from build123d import *

# Parameters (mm, degrees)
SKETCH2_R           = 7.62
BOSS_EXTRUDE2_DEPTH = 254
SKETCH3_R           = 5.08
CUT_EXTRUDE1_DEPTH  = 8.62


with BuildPart() as part:
    # Sketch2 → Boss-Extrude2 (new body)
    with BuildSketch(Plane(origin=(0, 0, 0), x_dir=(1, 0, 0), z_dir=(0, 1, 0))):
        Circle(SKETCH2_R)
    extrude(amount=BOSS_EXTRUDE2_DEPTH)

    # Sketch3 → Cut-Extrude1 (cut, through all)
    with BuildSketch(Plane(origin=(0, 0, 0), x_dir=(0, 0, -1), z_dir=(1, 0, 0))):
        with Locations((0, 157.537141192)):
            Circle(SKETCH3_R)
        with Locations((0, 81.337141192)):
            Circle(SKETCH3_R)
    extrude(amount=-CUT_EXTRUDE1_DEPTH, mode=Mode.SUBTRACT)


solid = part.part
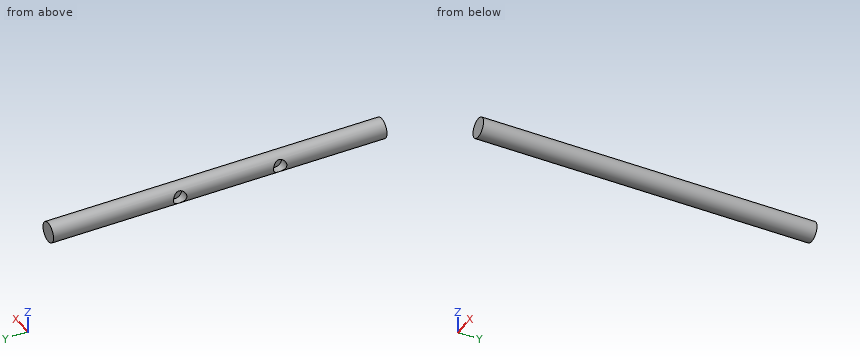
Check sheet for the modelled part. Datum: model origin and axes. Units: mm. Round coordinates to 2 decimals unless told otherwise and drop trailing zeros. Order: outer loops, then holes, each group sorted by start corner. A loop starts at its lowest first (then second) coordinate and runs counter-clockwise, first axis right, second up. Notation, with made-up numbers: M 61,72 L 67,72 A30 cw 67,101 Z; hole C 27,14.5 d8. An arc over 180 degrees is marked long. One line per item, written item: value. Start each with the question number.
1. Section check A-A on z = 0. Enter the section's corners in (x, y), and give its area (3 significant figures).
2. Section check C-C on x = 5. Enter the section's corners in (y, z), and give its area (3 significant figures).
3. Gauge pin test, flat ends, axial feed: P1, Ø8, axis at x = -5.5, y = 96.5, coming from the +Z side; P2, Ø6, axis at y = 157.54, z = 0, coming from the -X side; P3, Ø1, axis at x = -3.5, z = -1, coming from the -Y side; P4, Ø1, axis at y = 84, z = -4.5, coming from the -X side. Record the tip position at first contact, or that the pin passes through.
4. Section check B-B on y = 141.5. Enter the section's corners in (x, z), and give its area (3 significant figures).
5. Scan lines: line 1 along Y through (x, z) = (-4, 0); line 2 along Y through (x, z) = (-6, 1.75); line 3 along Z through (x, y) = (-3.25, 79). Record each from-to range of solid material in increasing order.
Results found:
1. outline: M -7.62,0 L 7.62,0 L 7.62,254 L -7.62,254 L -7.62,162.62 L 0,162.62 L 0,152.46 L -7.62,152.46 L -7.62,86.42 L 0,86.42 L 0,76.26 L -7.62,76.26 Z
1. area: 3,720 mm^2
2. outline: M 0,-5.75 L 254,-5.75 L 254,5.75 L 0,5.75 Z
2. area: 2,920 mm^2
3. P1: z = 7.47
3. P2: x = 0
3. P3: y = 0
3. P4: x = -6.41
4. outline: C 0,0 d15.24
4. area: 182 mm^2
5. line 1: 0 to 76.26, 86.42 to 152.46, 162.62 to 254
5. line 2: 0 to 76.57, 86.11 to 152.77, 162.31 to 254
5. line 3: -6.89 to -4.51, 4.51 to 6.89
